Autodesk Inventor part; units mm, degrees
ref_plane "YZ Plane" through (0, 0, 0) normal (1, 0, 0) x (0, 1, 0)
ref_plane "XZ Plane" through (0, 0, 0) normal (0, 1, 0) x (-1, 0, 0)
ref_plane "XY Plane" through (0, 0, 0) normal (0, 0, 1) x (1, 0, 0)
sketch "スケッチ1" plane through (0, 0, 0) normal (0, 0, 1) x (1, 0, 0)
  circle A0 centre (0, 0) radius 2.75
  dimension "d0" = 5.5
extrude "押し出し1" add sketch "スケッチ1" against normal blind 2.9
sketch "スケッチ2" plane through (0, 0, -2.9) normal (0, 0, -1) x (-1, 0, 0)
  circle A0 centre (0, 0) radius 1.5
  dimension "d3" = 3
extrude "押し出し2" add sketch "スケッチ2" along normal blind 6
thread "ねじ1"
fillet "フィレット1" radius 0.2 2 edges at (-2.75, 0, 0) (-2.75, 0, -2.9)
properties part number "M3×6ネジ" material "ステンレス鋼"
Source: CAD feature listing. Evaluate the final solid. Frame: model axes, mm. A direction names the side the tool comes from. Give positions to 0.01 mm unless a question says otherwise; leave off trailing zeros. Order: outer loops, then holes, each group sorted by start corner. A loop starts at its lowest first (then second) coordinate and runs counter-clockwise, first axis right, second up. Notation, with made-up numbers: (-6.75, 11.25) -> (3.25, 11.25) arc R24 cw to (3.25, 28.25) -> close; hole circle Ø11 at (1, 25.25). An arc over 180 degrees is marked (long way). Write item = value, one per line.
Q1. Material intervals for line 1 (Z direction, x = -0.85, y = -1.35); line 2 (X direction, y = 1.85, z = -1.75); line 3 (Y direction, x = 0.25, z = -1), sorted ascending. Write a range as from..to.
Data:
line_1 = -2.9..0
line_2 = -2.03..2.03
line_3 = -2.74..2.74
Q2. Set-up query: faces 1 (the face through (-0.596, -2.685, -1.432)), 2 (the face through (2, 0, -2.9)). Return all of +Z, -Z, +X, -X, +Y, -Y with unobstructed straight access to the full face (end or side cutting, diameter ignored); none if empty.
Data:
face_1 = +Z, -Z
face_2 = -Z
Q3. Cut plane D-D, the plane z = -7. Output: boundary loops of the cut face in (x, y), and give its area (3 significant figures).
Data:
outline = circle Ø3 at (0, 0)
area = 7.07 mm^2
Q4. Cut plane C-C, the plane z = -2. Output: boundary loops of the cut face in (x, y).
Data:
outline = circle Ø5.5 at (0, 0)
Q5. Cut plane A-A, the plane x = 0. Output: boundary loops of the cut face in (y, z), and give its area (3 significant figures).
Data:
outline = (-2.75, -2.7) arc R0.2 ccw to (-2.55, -2.9) -> (-1.5, -2.9) -> (-1.5, -8.9) -> (1.5, -8.9) -> (1.5, -2.9) -> (2.55, -2.9) arc R0.2 ccw to (2.75, -2.7) -> (2.75, -0.2) arc R0.2 ccw to (2.55, 0) -> (-2.55, 0) arc R0.2 ccw to (-2.75, -0.2) -> close
area = 33.9 mm^2
Q6. Pin query (flat end, axial travel): pin 1 (1 mm diameter, centred on x = -1.5, z = -6.5, fed in from -Y). Return the tip coordinate at first contact, or that it passes through.
Data:
pin_1 = -1.12
